from build123d import *

# Parameters (mm, degrees)
F0_R     = 19.05
F1_DEPTH = 20.32
F2_W     = 84.38881
F2_H     = 17.738584
F3_DEPTH = 43.18


with BuildPart() as f1:
    # F0 (on Right) → F1 (new body)
    with BuildSketch(Plane.YZ):
        with BuildLine():
            Line((-38.34097, 0), (-42.069936, 0))
            Line((-42.069936, 0), (-42.069936, -177.8))
            Line((-42.069936, -177.8), (42.318874, -177.8))
            Line((42.318874, -177.8), (42.318874, 0))
            Line((42.318874, 0), (38.34097, 0))
            ThreePointArc((38.34097, 0), (0, 38.34097), (-38.34097, 0))
        make_face()
        Circle(F0_R, mode=Mode.SUBTRACT)
    extrude(amount=F1_DEPTH)

    # F2 (on face) → F3 (join)
    with BuildSketch(Plane.YZ.offset(20.32)):
        with Locations((0.124469, -168.930708)):
            Rectangle(F2_W, F2_H)
    extrude(amount=F3_DEPTH)

    # F4: F1 across face


with BuildPart() as f1_1:
    add(f1.part)
    add(f1.part.mirror(Plane(origin=(63.5, 0.124469, -168.930708), x_dir=(0, 1, 0), z_dir=(1, 0, 0))))


solid = f1_1.part
Read the model definition and answer for the solid it produces. Units are mm, in the model's axes. A direction names the side the tool comes from. Round coordinates to 2 decimals unless told otherwise and drop trailing zeros. Order: outer loops, then holes, each group sorted by start corner. A loop starts at its lowest first (then second) coordinate and runs counter-clockwise, first axis right, second up.
1) Straight lines are drawn through the part: L1, parallel to X at y = -13.5, z = -90; L2, parallel to Z at x = 9, y = 0; L3, parallel to Z at x = 74.5, y = 25.5. For each, find the intervals that lie inside material, in ascending order.
2) The part is cut by section C-C on x = 118. Write down the section's boundary in (y, z).
3) Flat-ended cylindrical pins translate along their axes: pin 1 (1 mm diameter, centred on x = 75.5, y = -6, fed in from +Z); pin 2 (2 mm diameter, centred on x = 116, y = 39.5, fed in from +Z). Find the tip coordinate at first contact, or state that the pin passes through.
4) The mould has two halves that part along X. Classify faces 1 (the face through (64, 0, -160.061)), 2 (the face through (107, -42.07, -110)), 3 (the face through (127, 0, -68)), 4 (the face through (0, 0, -68)): released by +X, released by -X, zero draft, split by the parting line, or undercut.
5) The part is cut by section D-D on y = -11.5. Write down the section's boundary in (x, z).
6) The part is cut by section A-A on z = -61.5. Write down the section's boundary in (x, y).
7) For faces 5 (the face through (20.32, 0, -59)), 6 (the face through (116.98, 0.84, 38.33)), 7 (the face through (10, 40, 0)), determine the directions among +Z, -Z, +X, -X, +Y, -Y from which every point of the face is accessible in a straight line to the end or side of a thin tool.
8) The part is cut by section B-B on y = 0. Write down the section's boundary in (x, z).
Resolved:
1. L1: x = 0 to 20.32, 106.68 to 127
1. L2: z = -177.8 to -19.05, 19.05 to 38.34
1. L3: z = -177.8 to -160.06
2. outline: (-42.07, -177.8) - (42.32, -177.8) - (42.32, 0) - (38.34, 0) arc R38.34 ccw to (-38.34, 0) - (-42.07, 0) - close; hole circle Ø38.1 at (0, 0)
3. pin 1: stops at z = -160.06
3. pin 2: stops at z = 0
4. face 1: undercut
4. face 2: zero draft
4. face 3: released by +X
4. face 4: released by -X
5. outline: (0, -177.8) - (127, -177.8) - (127, -15.19) - (106.68, -15.19) - (106.68, -160.06) - (20.32, -160.06) - (20.32, -15.19) - (0, -15.19) - close; (0, 15.19) - (20.32, 15.19) - (20.32, 36.58) - (0, 36.58) - close; (106.68, 15.19) - (127, 15.19) - (127, 36.58) - (106.68, 36.58) - close
6. outline: (0, -42.07) - (20.32, -42.07) - (20.32, 42.32) - (0, 42.32) - close; (106.68, -42.07) - (127, -42.07) - (127, 42.32) - (106.68, 42.32) - close
7. face 5: +Z, +Y, -Y
7. face 6: +Z, +X, -X
7. face 7: +Z, +X, -X, +Y
8. outline: (0, -177.8) - (127, -177.8) - (127, -19.05) - (106.68, -19.05) - (106.68, -160.06) - (20.32, -160.06) - (20.32, -19.05) - (0, -19.05) - close; (0, 19.05) - (20.32, 19.05) - (20.32, 38.34) - (0, 38.34) - close; (106.68, 19.05) - (127, 19.05) - (127, 38.34) - (106.68, 38.34) - close
